```python
from build123d import *

# Parameters (mm, degrees)
SKETCH1_W               = 20
SKETCH1_H               = 25.4
BOSS_EXTRUDE1_DEPTH     = 80
SKETCH2_R               = 33.95
CUT_EXTRUDE1_DEPTH      = 80
CUT_EXTRUDE3_DEPTH      = 140.152703783
CUT_EXTRUDE3_DEPTH_BACK = 140.152703783
SKETCH3_W               = 10
SKETCH3_H               = 30.5


with BuildPart() as part:
    # Sketch1 → Boss-Extrude1 (new body)
    with BuildSketch(Plane(origin=(0, 0, 0), x_dir=(1, 0, 0), z_dir=(0, 1, 0))):
        with BuildLine():
            Line((-17.528898419, 17.5), (17.528898419, 17.5))
            ThreePointArc((17.528898419, 17.5), (85.182138113, 0), (17.528898419, -17.5))
            Line((17.528898419, -17.5), (-17.528898419, -17.5))
            ThreePointArc((-17.528898419, -17.5), (-85.182138113, 0), (-17.528898419, 17.5))
        make_face()
        with Locations((-92.873761816, 0)):
            Rectangle(SKETCH1_W, SKETCH1_H)
        with Locations((92.873761816, 0)):
            Rectangle(SKETCH1_W, SKETCH1_H)
    extrude(amount=BOSS_EXTRUDE1_DEPTH)

    # Sketch2 → Cut-Extrude1 (cut)
    with BuildSketch(Plane(origin=(0, 80, 0), x_dir=(1, 0, 0), z_dir=(0, 1, 0))):
        with Locations(Location((-49.108204523, 0, 0), (0, 0, 270))):
            Circle(SKETCH2_R)
        with Locations(Location((49.092138113, 0, 0), (0, 0, 270))):
            Circle(SKETCH2_R)
    extrude(amount=-CUT_EXTRUDE1_DEPTH, mode=Mode.SUBTRACT)

    # Sketch3 → Cut-Extrude3 (cut, two sides: drawn at the far end of the back side and taken through both)
    with BuildSketch(Plane.XY.offset(12.7).offset(-CUT_EXTRUDE3_DEPTH_BACK)):
        with Locations((0, 40)):
            Rectangle(SKETCH3_W, SKETCH3_H)
        with Locations((-94.873761816, 40)):
            Rectangle(SKETCH3_W, SKETCH3_H)
        with Locations((94.873761816, 40)):
            Rectangle(SKETCH3_W, SKETCH3_H)
    extrude(amount=CUT_EXTRUDE3_DEPTH + CUT_EXTRUDE3_DEPTH_BACK, mode=Mode.SUBTRACT)


solid = part.part
```
Read the model definition and answer for the solid it produces. Units are mm, in the model's axes. A direction names the side the tool comes from. Give positions to 0.01 mm unless a question says otherwise; leave off trailing zeros. Order: outer loops, then holes, each group sorted by start corner. A loop starts at its lowest first (then second) coordinate and runs counter-clockwise, first axis right, second up. Notation, with made-up numbers: (-14.5, -4) -> (-1.5, -4) arc R21 ccw to (-1.5, 7) -> close; hole circle Ø9 at (-5, 80.5). An arc over 180 degrees is marked (long way). One line per item, written item: value. Start each with the question number.
(1) The part is cut by section C-C (y = 49). Determine the outline of the cut face in (x, z), and give its area (3 significant figures).
(2) For a pull along Y with two mould halves and no side action, classify faces 4 (the flat face through (99.874, 40, 0)), 5 (the flat face through (-5, 40, 0)), 6 (the flat face through (0, 0, 0)), 7 (the cylindrical face through (-51.16, 39.44, 36.03)) as released by +Y, released by -Y, zero draft, split by the parting line, or undercut.
(3) The part is cut by section A-A (z = 0). Determine the outline of the cut face in (x, y), and give its area (3 significant figures).
(4) The part is cut by section B-B (x = 78). Determine the outline of the cut face in (y, z).
(5) The part is cut by section D-D (y = 8.5). Determine the outline of the cut face in (x, z), and give its area (3 significant figures).
(6) Flat-ended cylindrical pins translate along their axes: P1, Ø6, axis at x = -91.5, y = 46.5, coming from the +Z side; P2, Ø12, axis at x = -67, y = 70, coming from the -Z side; P3, Ø8, axis at y = 69, z = 28.5, coming from the -X side; P4, Ø10, axis at x = 35, z = 23.5, coming from the -Y side. Find the tip coordinate at first contact, or state that the pin passes through.
(7) A tool of negligible diameter and unlimited length cuts with its end or side. For faces 1 (the flat face through (-8, 39, 17.5)), 2 (the flat face through (-89, 39, 12.7)), 3 (the flat face through (95, 24.75, 0)), from which of +Z, -Z, +X, -X, +Y, -Y can it reach the whole face along a straight path? Write none if from no direction.
(8) Straight lines are drawn through the part: L1, parallel to X at y = 50, z = 0; L2, parallel to X at y = 19, z = 0; L3, parallel to X at y = 7, z = -11.5. For each, find the intervals that lie inside material, in ascending order.
Taken from the geometry:
1. outline: (-102.87, -12.7) -> (-99.87, -12.7) -> (-99.87, 12.7) -> (-102.87, 12.7) -> close; (-89.87, -12.7) -> (-82.87, -12.7) arc R36.09 ccw to (-17.53, -17.5) -> (-5, -17.5) -> (-5, 17.5) -> (-17.53, 17.5) arc R36.09 ccw to (-82.87, 12.7) -> (-89.87, 12.7) -> close; (5, -17.5) -> (17.53, -17.5) arc R36.09 ccw to (82.87, -12.7) -> (89.87, -12.7) -> (89.87, 12.7) -> (82.87, 12.7) arc R36.09 ccw to (17.53, 17.5) -> (5, 17.5) -> close; (99.87, -12.7) -> (102.87, -12.7) -> (102.87, 12.7) -> (99.87, 12.7) -> close; hole circle Ø67.9 at (-49.11, 0); hole circle Ø67.9 at (49.09, 0)
1. area: 2,030 mm^2
2. face 4: undercut
2. face 5: undercut
2. face 6: released by -Y
2. face 7: zero draft
3. outline: (-102.87, 0) -> (-83.06, 0) -> (-83.06, 80) -> (-102.87, 80) -> close; (-15.16, 0) -> (15.14, 0) -> (15.14, 80) -> (-15.16, 80) -> close; (83.04, 0) -> (102.87, 0) -> (102.87, 80) -> (83.04, 80) -> close; hole (-99.87, 24.75) -> (-89.87, 24.75) -> (-89.87, 55.25) -> (-99.87, 55.25) -> close; hole (-5, 24.75) -> (5, 24.75) -> (5, 55.25) -> (-5, 55.25) -> close; hole (89.87, 24.75) -> (99.87, 24.75) -> (99.87, 55.25) -> (89.87, 55.25) -> close
3. area: 4,680 mm^2
4. outline: (0, -21.61) -> (80, -21.61) -> (80, -17.8) -> (0, -17.8) -> close; (0, 17.8) -> (80, 17.8) -> (80, 21.61) -> (0, 21.61) -> close
5. outline: (-102.87, -12.7) -> (-82.87, -12.7) arc R36.09 ccw to (-17.53, -17.5) -> (17.53, -17.5) arc R36.09 ccw to (82.87, -12.7) -> (102.87, -12.7) -> (102.87, 12.7) -> (82.87, 12.7) arc R36.09 ccw to (17.53, 17.5) -> (-17.53, 17.5) arc R36.09 ccw to (-82.87, 12.7) -> (-102.87, 12.7) -> close; hole circle Ø67.9 at (-49.11, 0); hole circle Ø67.9 at (49.09, 0)
5. area: 2,890 mm^2
6. P1: z = 12.7
6. P2: z = -34.07
6. P3: x = -75.59
6. P4: through
7. face 1: +Z, +Y, -Y
7. face 2: +Z, -X, +Y, -Y
7. face 3: +Z, -Z
8. L1: -102.87 to -99.87, -89.87 to -83.06, -15.16 to -5, 5 to 15.14, 83.04 to 89.87, 99.87 to 102.87
8. L2: -102.87 to -83.06, -15.16 to 15.14, 83.04 to 102.87
8. L3: -102.87 to -81.05, -17.17 to 17.15, 81.04 to 102.87
